Part print with two shaded views. Sizes in mm from the minimum x, y, z corner. Round coordinates to 2 decimals unless told otherwise and drop trailing zeros. Loops run counter-clockwise (first coordinate to the right, second up) from the corner with the lowest first, then second, coordinate; pieces in that order, holes last. Notation, with made-up numbers: (9, 12) - (49, 12) arc R19 cw to (49, 23) - close; hole circle Ø5 at (-24.5, 72.25). An arc over 180 degrees is marked (long way). Write each question's results on one line, items separated by ' | '. Start each with the question number.
(1) Flat gauge pins, fed straight in: P1, Ø1.8, axis at x = 168, y = 4.5, coming from the +Z side; P2, Ø1.8, axis at y = 1.5, z = 13.5, coming from the -X side; P3, Ø1, axis at x = 35, y = 4, coming from the -Z side. Where does each tip first touch, or does it go through?
(2) Cut at A-A, the plane z = 13.5. List the corners of the cut face in (x, y) (1 decimal).
(3) Cut at C-C, the plane x = 69. List the corners of the cut face in (y, z).
(4) Drill centre lines: L1, parallel to X at y = 5.3, z = 12.5 (1 decimal); L2, parallel to Z at x = 163.5, y = 1.55. Where is each one in solid material? Low to high.
(5) Cut at B-B, the plane y = 2.3. List the corners of the cut face in (x, z) (1 decimal).
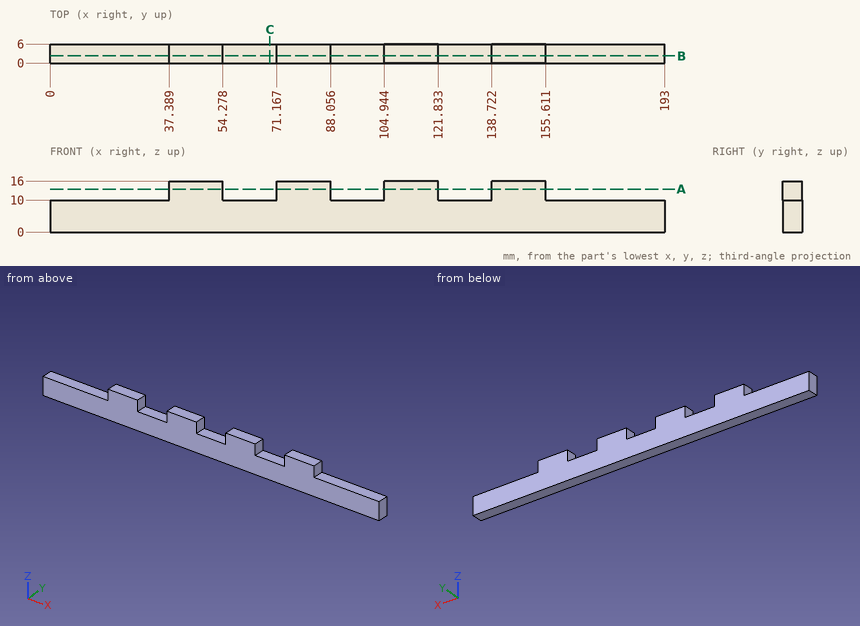
A:
1) P1: z = 10 | P2: x = 37.39 | P3: z = 0
2) outline: (37.4, 0) - (54.3, 0) - (54.3, 6) - (37.4, 6) - close; (71.2, 0) - (88.1, 0) - (88.1, 6) - (71.2, 6) - close; (104.9, 0) - (121.8, 0) - (121.8, 6) - (104.9, 6) - close; (138.7, 0) - (155.6, 0) - (155.6, 6) - (138.7, 6) - close
3) outline: (0, 0) - (6, 0) - (6, 10) - (0, 10) - close
4) L1: 37.4 to 54.3, 71.2 to 88.1, 104.9 to 121.8, 138.7 to 155.6 | L2: 0 to 10
5) outline: (0, 0) - (193, 0) - (193, 10) - (155.6, 10) - (155.6, 16) - (138.7, 16) - (138.7, 10) - (121.8, 10) - (121.8, 16) - (104.9, 16) - (104.9, 10) - (88.1, 10) - (88.1, 16) - (71.2, 16) - (71.2, 10) - (54.3, 10) - (54.3, 16) - (37.4, 16) - (37.4, 10) - (0, 10) - close
